Input: part model. Units: mm. Frame: model coordinates. A direction names the side the tool comes from. Round coordinates to 2 decimals unless told otherwise and drop trailing zeros. Loops run counter-clockwise (first coordinate to the right, second up) from the corner with the lowest first, then second, coordinate; pieces in that order, holes last. Notation, with made-up numbers: M -6.75,-4.75 L 21.25,-4.75 A28 ccw 21.25,24.25 Z; hole C 33.25,81.25 d11. An arc over 180 degrees is marked long. Return JSON: item names as keys, results as strings. Group by question number.
1) Material intervals for line 1 (X direction, y = 1.45, z = 14); line 2 (X direction, y = 5.75, z = -10); line 3 (Y direction, x = -10, z = -7), sorted ascending. Write a range as from..to.
2) Section C-C (y = 2.75). Output: boundary loops of the cut face in (x, z).
3) Mould query, pull axis X, two halves, no side actions, for faces 1 (the face through (0.03, 5.7, 9.25)), 2 (the face through (-2.5, 6, -9)), 3 (the face through (4, 9.5, -7)). Classes: +X half, -X half, draft (parallel to the pull), parting line (faces both ways), or undercut.
4) Section A-A (x = 14). Output: boundary loops of the cut face in (y, z).
5) Access query for faces 4 (the face through (1.802, 17.458, 5.723)), 5 (the face through (0.1, 5.7, 12.5)), 6 (the face through (-6.834, 22.472, -1.517)), 7 (the face through (-6, 6, -8.5)). Directions: +Z, -Z, +X, -X, +Y, -Y. A direction counts if a zero-diameter tool reaches every point of the face in a straight line with its end or side. Return the directions, or none.
6) Contact query for flat-ended pins moving along their axis: P1, Ø3, axis at y = 9, z = -11.5, coming from the +X side; P2, Ø6.5, axis at x = 5.5, y = 6.5, coming from the -Z side; P3, Ø3, axis at x = -3, y = 20, coming from the -Z side; P4, Ø1, axis at y = 15, z = -10, coming from the -X side. Output: stop coordinate, or through.
7) Section B-B (z = 14). Output: boundary loops of the cut face in (x, y), plus the area to 3 significant figures.
8) Section D-D (x = 0). Output: boundary loops of the cut face in (y, z), plus the area to 4 significant figures.
from build123d import *

# Parameters (mm, degrees)
SKETCH_1_W      = 32
SKETCH_1_H      = 32
SKETCH_1_R      = 1.25
EXTRUDE_1_DEPTH = 2
SKETCH_2_R      = 0.75
EXTRUDE_2_DEPTH = 7.5
SKETCH_3_R      = 7.75
EXTRUDE_3_DEPTH = 5
SKETCH_4_R      = 6
EXTRUDE_4_DEPTH = 6
SKETCH_5_R      = 7
EXTRUDE_5_DEPTH = 4


with BuildPart() as part:
    # 草图1 → 凸台-拉伸1 (new body)
    with BuildSketch(Plane(origin=(0, 0, 0), x_dir=(1, 0, 0), z_dir=(0, 1, 0))):
        Rectangle(SKETCH_1_W, SKETCH_1_H)
        with Locations(Location((-14, 14, 0), (0, 0, 270))):
            Circle(SKETCH_1_R, mode=Mode.SUBTRACT)
        with Locations(Location((14, 14, 0), (0, 0, 270))):
            Circle(SKETCH_1_R, mode=Mode.SUBTRACT)
        with Locations(Location((14, -14, 0), (0, 0, 270))):
            Circle(SKETCH_1_R, mode=Mode.SUBTRACT)
        with Locations(Location((-14, -14, 0), (0, 0, 270))):
            Circle(SKETCH_1_R, mode=Mode.SUBTRACT)
    extrude(amount=EXTRUDE_1_DEPTH)

    # 草图2 → 凸台-拉伸2 (add)
    with BuildSketch(Plane(origin=(0, 2, 0), x_dir=(1, 0, 0), z_dir=(0, 1, 0))):
        with BuildLine():
            Line((-2.5, -10), (-2.5, -8.5))
            Line((-2.5, -8.5), (-8.5, -8.5))
            Line((-8.5, -8.5), (-8.5, 8.5))
            Line((-8.5, 8.5), (-2.5, 8.5))
            Line((-2.5, 8.5), (-2.5, 10))
            ThreePointArc((-2.5, 10), (0, 12.5), (2.5, 10))
            Line((2.5, 10), (2.5, 8.5))
            Line((2.5, 8.5), (8.5, 8.5))
            Line((8.5, 8.5), (8.5, -8.5))
            Line((8.5, -8.5), (2.5, -8.5))
            Line((2.5, -8.5), (2.5, -10))
            ThreePointArc((2.5, -10), (0, -12.5), (-2.5, -10))
        make_face()
        with Locations(Location((0, 10, 0), (0, 0, 270))):
            Circle(SKETCH_2_R, mode=Mode.SUBTRACT)
        with Locations(Location((0, -10, 0), (0, 0, 270))):
            Circle(SKETCH_2_R, mode=Mode.SUBTRACT)
    extrude(amount=EXTRUDE_2_DEPTH)

    # 草图3 → 凸台-拉伸3 (add)
    with BuildSketch(Plane(origin=(0, 9.5, 0), x_dir=(1, 0, 0), z_dir=(0, 1, 0))):
        with Locations(Location((0, 0, 0), (0, 0, 270))):
            Circle(SKETCH_3_R)
    extrude(amount=EXTRUDE_3_DEPTH)

    # 草图4 → 凸台-拉伸4 (add)
    with BuildSketch(Plane(origin=(0, 14.5, 0), x_dir=(1, 0, 0), z_dir=(0, 1, 0))):
        with Locations(Location((0, 0, 0), (0, 0, 270))):
            Circle(SKETCH_4_R)
    extrude(amount=EXTRUDE_4_DEPTH)

    # 草图5 → 凸台-拉伸5 (add)
    with BuildSketch(Plane(origin=(0, 20.5, 0), x_dir=(1, 0, 0), z_dir=(0, 1, 0))):
        with Locations(Location((0, 0, 0), (0, 0, 270))):
            Circle(SKETCH_5_R)
    extrude(amount=EXTRUDE_5_DEPTH)


solid = part.part
Returned:
{
 "1": {"line 1": "x = -16..-15.25, -12.75..12.75, 15.25..16", "line 2": "x = -2.5..-0.75, 0.75..2.5", "line 3": "y = 0..2"},
 "2": {"outline": "M -8.5,-8.5 L -2.5,-8.5 L -2.5,-10 A2.5 ccw 2.5,-10 L 2.5,-8.5 L 8.5,-8.5 L 8.5,8.5 L 2.5,8.5 L 2.5,10 A2.5 ccw -2.5,10 L -2.5,8.5 L -8.5,8.5 Z; hole C 0,-10 d1.5; hole C 0,10 d1.5"},
 "3": {"face 1": "undercut", "face 2": "-X half", "face 3": "draft"},
 "4": {"outline": "M 0,-16 L 2,-16 L 2,-15.25 L 0,-15.25 Z; M 0,-12.75 L 2,-12.75 L 2,12.75 L 0,12.75 Z; M 0,15.25 L 2,15.25 L 2,16 L 0,16 Z"},
 "5": {"face 4": "none", "face 5": "+Z, +Y", "face 6": "+Y", "face 7": "-Z, -X, +Y"},
 "6": {"P1": "stops at x = 2.5", "P2": "stops at z = -11.09", "P3": "stops at z = -6.82", "P4": "passes through"},
 "7": {"outline": "M -16,0 L -15.25,0 L -15.25,2 L -16,2 Z; M -12.75,0 L 12.75,0 L 12.75,2 L -12.75,2 Z; M 15.25,0 L 16,0 L 16,2 L 15.25,2 Z", "area": "54.0 mm^2"},
 "8": {"outline": "M 0,-16 L 2,-16 L 2,-12.5 L 9.5,-12.5 L 9.5,-10.75 L 2,-10.75 L 2,-9.25 L 9.5,-9.25 L 9.5,-7.75 L 14.5,-7.75 L 14.5,-6 L 20.5,-6 L 20.5,-7 L 24.5,-7 L 24.5,7 L 20.5,7 L 20.5,6 L 14.5,6 L 14.5,7.75 L 9.5,7.75 L 9.5,9.25 L 2,9.25 L 2,10.75 L 9.5,10.75 L 9.5,12.5 L 2,12.5 L 2,16 L 0,16 Z", "area": "434.5 mm^2"}
}
